```python
from build123d import *

# Parameters (mm, degrees)
SKETCH1_W           = 38
SKETCH1_H           = 5
SKETCH1_W_2         = 10
SKETCH1_H_2         = 2.5
BOSS_EXTRUDE1_DEPTH = 1.25


with BuildPart() as part:
    # Sketch1 → Boss-Extrude1 (new, symmetric)
    with BuildSketch(Plane.XY):
        Polygon((-75, 6.25), (-75, 2.5), (-67, 2.5), (-67, -2.5), (-75, -2.5), (-75, -6.25), (-67, -6.25), (-67, -11.25), (-75, -11.25), (-75, -16.25), (-67, -16.25), (-67, -18.75), (-75, -18.75), (-75, -21.25), (75, -21.25), (75, -18.75), (67, -18.75), (67, -16.25), (75, -16.25), (75, -11.25), (67, -11.25), (67, -6.25), (75, -6.25), (75, -2.5), (67, -2.5), (67, 2.5), (75, 2.5), (75, 6.25), (67, 6.25), (67, 11.25), (75, 11.25), (75, 16.25), (67, 16.25), (67, 18.75), (75, 18.75), (75, 21.25), (-75, 21.25), (-75, 18.75), (-67, 18.75), (-67, 16.25), (-75, 16.25), (-75, 11.25), (-67, 11.25), (-67, 6.25), align=None)
        with Locations((0, 8.75)):
            Rectangle(SKETCH1_W, SKETCH1_H, mode=Mode.SUBTRACT)
        Rectangle(SKETCH1_W, SKETCH1_H, mode=Mode.SUBTRACT)
        with Locations((0, -17.5)):
            Rectangle(SKETCH1_W_2, SKETCH1_H_2, mode=Mode.SUBTRACT)
        with Locations((0, 17.5)):
            Rectangle(SKETCH1_W_2, SKETCH1_H_2, mode=Mode.SUBTRACT)
        with Locations((20, 17.5)):
            Rectangle(SKETCH1_W_2, SKETCH1_H_2, mode=Mode.SUBTRACT)
        with Locations((20, -17.5)):
            Rectangle(SKETCH1_W_2, SKETCH1_H_2, mode=Mode.SUBTRACT)
        with Locations((40, 17.5)):
            Rectangle(SKETCH1_W_2, SKETCH1_H_2, mode=Mode.SUBTRACT)
        with Locations((40, -17.5)):
            Rectangle(SKETCH1_W_2, SKETCH1_H_2, mode=Mode.SUBTRACT)
        with Locations((60, 17.5)):
            Rectangle(SKETCH1_W_2, SKETCH1_H_2, mode=Mode.SUBTRACT)
        with Locations((60, -17.5)):
            Rectangle(SKETCH1_W_2, SKETCH1_H_2, mode=Mode.SUBTRACT)
        with Locations((-20, -17.5)):
            Rectangle(SKETCH1_W_2, SKETCH1_H_2, mode=Mode.SUBTRACT)
        with Locations((-20, 17.5)):
            Rectangle(SKETCH1_W_2, SKETCH1_H_2, mode=Mode.SUBTRACT)
        with Locations((-40, -17.5)):
            Rectangle(SKETCH1_W_2, SKETCH1_H_2, mode=Mode.SUBTRACT)
        with Locations((-40, 17.5)):
            Rectangle(SKETCH1_W_2, SKETCH1_H_2, mode=Mode.SUBTRACT)
        with Locations((-60, -17.5)):
            Rectangle(SKETCH1_W_2, SKETCH1_H_2, mode=Mode.SUBTRACT)
        with Locations((-60, 17.5)):
            Rectangle(SKETCH1_W_2, SKETCH1_H_2, mode=Mode.SUBTRACT)
        with Locations((0, -8.75)):
            Rectangle(SKETCH1_W, SKETCH1_H, mode=Mode.SUBTRACT)
        with Locations((-46, 0)):
            Rectangle(SKETCH1_W, SKETCH1_H, mode=Mode.SUBTRACT)
        with Locations((-46, 8.75)):
            Rectangle(SKETCH1_W, SKETCH1_H, mode=Mode.SUBTRACT)
        with Locations((-46, -8.75)):
            Rectangle(SKETCH1_W, SKETCH1_H, mode=Mode.SUBTRACT)
        with Locations((46, 8.75)):
            Rectangle(SKETCH1_W, SKETCH1_H, mode=Mode.SUBTRACT)
        with Locations((46, 0)):
            Rectangle(SKETCH1_W, SKETCH1_H, mode=Mode.SUBTRACT)
        with Locations((46, -8.75)):
            Rectangle(SKETCH1_W, SKETCH1_H, mode=Mode.SUBTRACT)
    extrude(amount=BOSS_EXTRUDE1_DEPTH, both=True)


solid = part.part
```
Input: part model. Units: mm. Frame: model coordinates. A direction names the side the tool comes from. Give positions to 0.01 mm unless a question says otherwise; leave off trailing zeros. Write each loop counter-clockwise with the first axis right and the second up, starting at its lowest first coordinate (ties: lowest second). Pieces come first, ordered by that corner, then holes. Notation, with made-up numbers: (-17.75, 23) - (22.25, 23) arc R15 cw to (22.25, 49) - close; hole circle Ø4 at (71, -9). An arc over 180 degrees is marked (long way). Write item = value, one per line. Start each with the question number.
1. Section query B-B, the plane y = -1. Output: boundary loops of the cut face in (x, z).
2. Section query D-D, the plane x = -42. Output: boundary loops of the cut face in (y, z).
3. Section query C-C, the plane x = -21. Output: boundary loops of the cut face in (y, z).
4. Access query for faces 1 (the flat face through (-67, -17, 0)), 2 (the flat face through (15, -18, 0)). Directions: +Z, -Z, +X, -X, +Y, -Y. A direction counts if a zero-diameter tool reaches every point of the face in a straight line with its end or side. Return the directions, or none.
5. Ray query, L1, parallel to X at y = -11, z = -0.2; L2, parallel to Y at x = 61.5, z = 0.6; L3, parallel to Y at x = -52.5, z = 0.75. Return the intervals inside material, ascending.
6. First-contact query: pin 1 Ø0.8 at (y, z) = (1, -0.5) entering from -X; pin 2 Ø0.8 at (y, z) = (8.5, 0) entering from +X. Flat tips, straight axial feed; report the tip coordinate or a pass-through.
7. Section query A-A, the plane x = 12.5. Output: boundary loops of the cut face in (y, z).
Check sheet entries:
q1.outline = (-67, -1.25) - (-65, -1.25) - (-65, 1.25) - (-67, 1.25) - close; (-27, -1.25) - (-19, -1.25) - (-19, 1.25) - (-27, 1.25) - close; (19, -1.25) - (27, -1.25) - (27, 1.25) - (19, 1.25) - close; (65, -1.25) - (67, -1.25) - (67, 1.25) - (65, 1.25) - close
q2.outline = (-21.25, -1.25) - (-18.75, -1.25) - (-18.75, 1.25) - (-21.25, 1.25) - close; (-16.25, -1.25) - (-11.25, -1.25) - (-11.25, 1.25) - (-16.25, 1.25) - close; (-6.25, -1.25) - (-2.5, -1.25) - (-2.5, 1.25) - (-6.25, 1.25) - close; (2.5, -1.25) - (6.25, -1.25) - (6.25, 1.25) - (2.5, 1.25) - close; (11.25, -1.25) - (16.25, -1.25) - (16.25, 1.25) - (11.25, 1.25) - close; (18.75, -1.25) - (21.25, -1.25) - (21.25, 1.25) - (18.75, 1.25) - close
q3.outline = (-21.25, -1.25) - (-18.75, -1.25) - (-18.75, 1.25) - (-21.25, 1.25) - close; (-16.25, -1.25) - (16.25, -1.25) - (16.25, 1.25) - (-16.25, 1.25) - close; (18.75, -1.25) - (21.25, -1.25) - (21.25, 1.25) - (18.75, 1.25) - close
q4.face_1 = +Z, -Z, -X
q4.face_2 = +Z, -Z
q5.L1 = -67 to -65, -27 to -19, 19 to 27, 65 to 67
q5.L2 = -21.25 to -18.75, -16.25 to -11.25, -6.25 to -2.5, 2.5 to 6.25, 11.25 to 16.25, 18.75 to 21.25
q5.L3 = -21.25 to -11.25, -6.25 to -2.5, 2.5 to 6.25, 11.25 to 21.25
q6.pin_1 = -67
q6.pin_2 = 67
q7.outline = (-21.25, -1.25) - (-11.25, -1.25) - (-11.25, 1.25) - (-21.25, 1.25) - close; (-6.25, -1.25) - (-2.5, -1.25) - (-2.5, 1.25) - (-6.25, 1.25) - close; (2.5, -1.25) - (6.25, -1.25) - (6.25, 1.25) - (2.5, 1.25) - close; (11.25, -1.25) - (21.25, -1.25) - (21.25, 1.25) - (11.25, 1.25) - close
